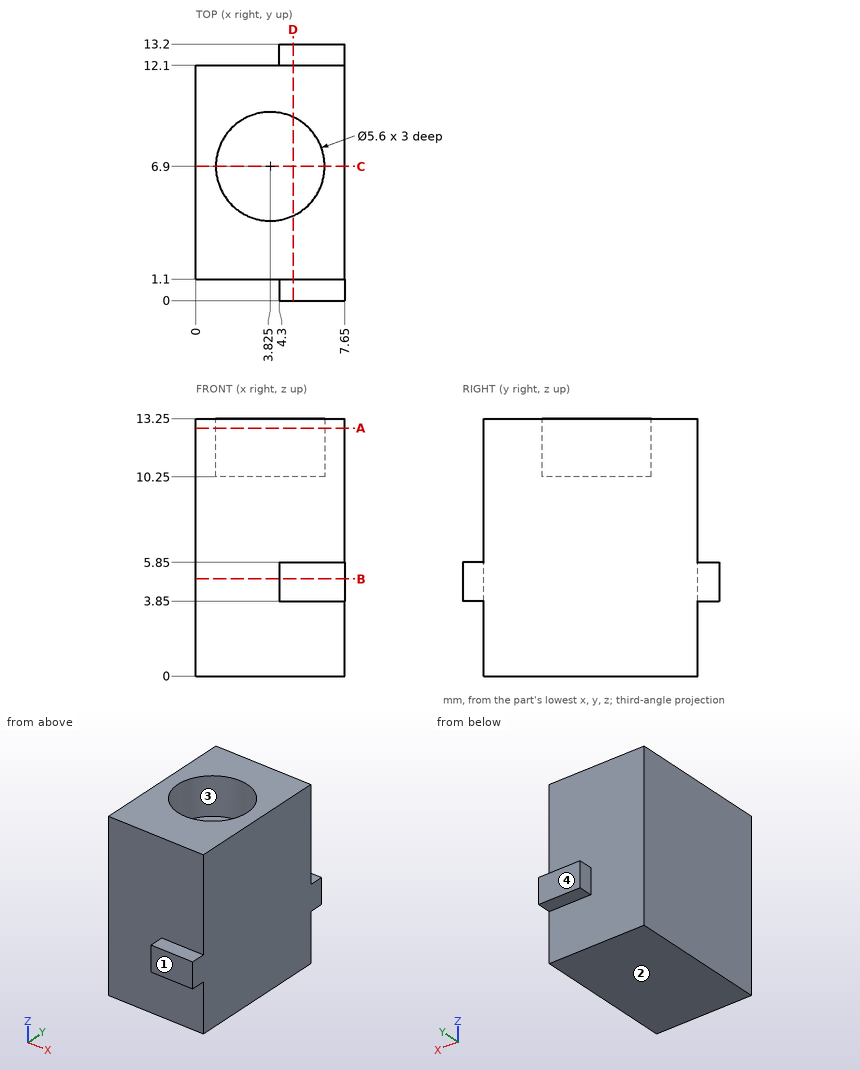
The figure shows three views and two pictorial views of one solid part (mm, origin at its lowest corner). Answer the questions. Give positions to 0.01 mm unless a question says otherwise; leave off trailing zeros. Loops run counter-clockwise (first coordinate to the right, second up) from the corner with the lowest first, then second, coordinate; pieces in that order, holes last. Notation, with made-up numbers: (51.25, -20.5) -> (84.25, -20.5) arc R21 cw to (84.25, 2.5) -> close; hole circle Ø1 at (-18, -8.75). An arc over 180 degrees is marked (long way). Put each result on its own line as item: value. Start each with the question number.
Item 1: The mould has two halves that part along Y. Classify the marked faces 1, 2, 3 and 4: released by +Y, released by -Y, zero draft, split by the parting line, or undercut.
Item 2: The part is cut by section C-C (y = 6.9). Give the vertices of the cut face in (x, z) (3 decimals), then the cut area to 3 significant figures.
Item 3: The part is cut by section D-D (x = 5). Give the vertices of the cut face in (y, z).
Item 4: Find the intervals of material crossed by L1, parallel to Z at x = 4.5, y = 0.5; L2, parallel to Z at x = 4.5, y = 6; L3, parallel to Y at x = 6.75, z = 2.75, in increasing order. Write a range as [from, to].
Item 5: Each of these flat-tipped pins is pushed along its axis until it touches: P1, Ø3, axis at x = 2.5, z = 5, coming from the +Y side; P2, Ø4, axis at x = 2, z = 7, coming from the -Y side; P3, Ø0.6, axis at y = 0.5, z = 4.5, coming from the -X side. Where does it stop, or does it pass through?
Item 6: The part is cut by section A-A (z = 12.75). Give the vertices of the cut face in (x, y) (3 decimals), then the cut area to 3 significant figures.
Item 7: The part is cut by section B-B (z = 5). Give the vertices of the cut face in (x, y).
Answers below:
1. face 1: released by -Y
1. face 2: zero draft
1. face 3: undercut
1. face 4: released by +Y
2. outline: (0, 0) -> (7.65, 0) -> (7.65, 13.25) -> (6.625, 13.25) -> (6.625, 10.25) -> (1.025, 10.25) -> (1.025, 13.25) -> (0, 13.25) -> close
2. area: 84.6 mm2
3. outline: (0, 3.85) -> (1.1, 3.85) -> (1.1, 0) -> (12.1, 0) -> (12.1, 3.85) -> (13.2, 3.85) -> (13.2, 5.85) -> (12.1, 5.85) -> (12.1, 13.25) -> (9.44, 13.25) -> (9.44, 10.25) -> (4.36, 10.25) -> (4.36, 13.25) -> (1.1, 13.25) -> (1.1, 5.85) -> (0, 5.85) -> close
4. L1: [3.85, 5.85]
4. L2: [0, 10.25]
4. L3: [1.1, 12.1]
5. P1: y = 12.1
5. P2: y = 1.1
5. P3: x = 4.3
6. outline: (0, 1.1) -> (7.65, 1.1) -> (7.65, 12.1) -> (0, 12.1) -> close; hole circle Ø5.6 at (3.825, 6.9)
6. area: 59.5 mm2
7. outline: (0, 1.1) -> (4.3, 1.1) -> (4.3, 0) -> (7.65, 0) -> (7.65, 13.2) -> (4.3, 13.2) -> (4.3, 12.1) -> (0, 12.1) -> close
